Answer from the drawing. Dimensions are ordinates in mm from the lowest x, y and z of the part. A direction names the side the tool comes from. Give positions to 0.01 mm unless a question says otherwise; leave off trailing zeros. Order: outer loops, then holes, each group sorted by start corner. A loop starts at its lowest first (then second) coordinate and runs counter-clockwise, first axis right, second up. Notation, with made-up numbers: (49, 60) - (87, 60) arc R20 ccw to (87, 68) - close; hole circle Ø4 at (89.5, 88). An arc over 180 degrees is marked (long way). Use a Markdown table: item, result. Add a question column.
1) Find section D-D, the plane y = 87. Determine the outline of the cut face in (x, z).
2) Flat-ended cylindrical pins translate along their axes: pin 1 (5.5 mm diameter, centred on y = 111.5, z = 12, fed in from +X); pin 2 (9 mm diameter, centred on x = 9, y = 117, fed in from -Z); pin 3 (4 mm diameter, centred on x = 4.5, z = 4, fed in from +Y). Find the tip coordinate at first contact, or state that the pin passes through.
3) Find section B-B, the plane x = 10. Determine the outline of the cut face in (y, z).
4) Straight lines are drawn through the part: line 1 (Y direction, x = 1, z = 10); line 2 (Z direction, x = 0.75, y = 10). For each, find the intervals that lie inside material, in ascending order.
5) For the marked faces 1 and 2, determine the directions among +Z, -Z, +X, -X, +Y, -Y from which every point of the face is accessible in a straight line to the end or side of a thin tool.
6) Find section C-C, the plane z = 10. Determine the outline of the cut face in (x, y).
7) Find section A-A, the plane y = 10. Determine the outline of the cut face in (x, z), plus the area to 4 significant figures.
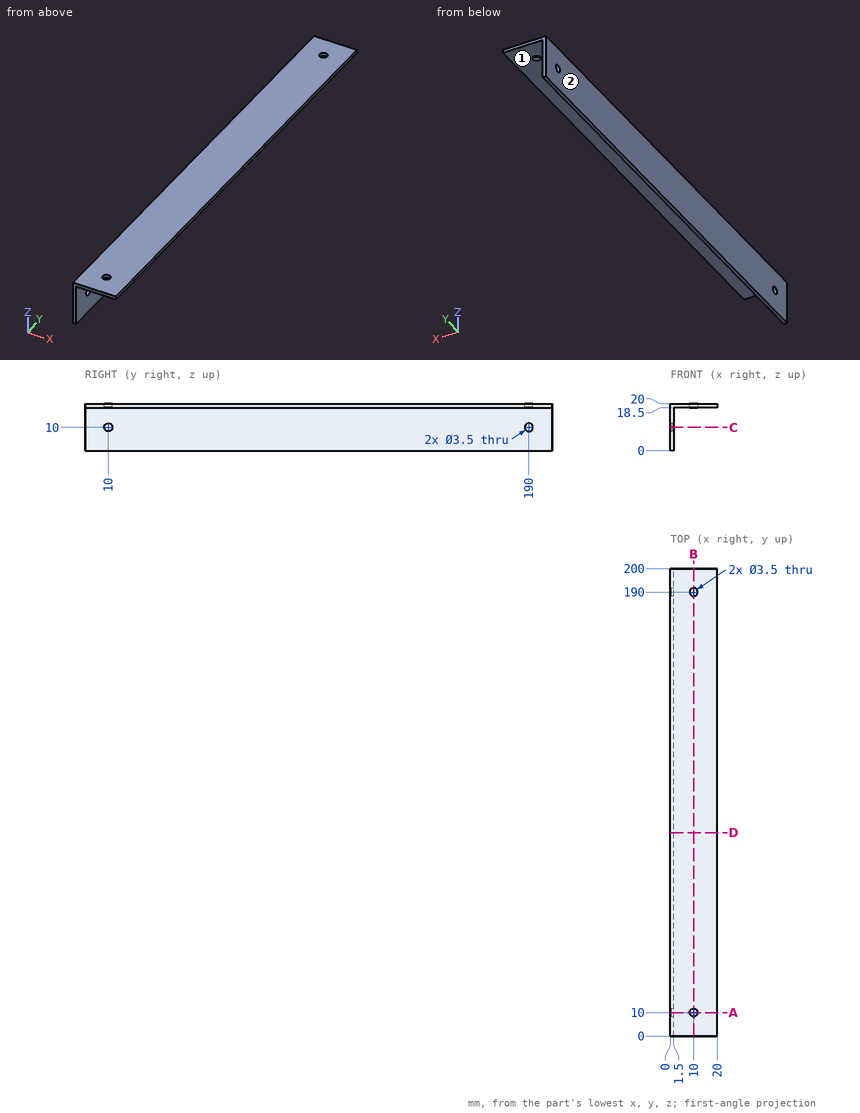
The answers:
| question | item | result |
|---|---|---|
| 1 | outline | (0, 0) - (1.5, 0) - (1.5, 18.5) - (20, 18.5) - (20, 20) - (0, 20) - close |
| 2 | pin 1 | x = 1.5 |
| 2 | pin 2 | z = 18.5 |
| 2 | pin 3 | through |
| 3 | outline | (0, 18.5) - (8.25, 18.5) - (8.25, 20) - (0, 20) - close; (11.75, 18.5) - (188.25, 18.5) - (188.25, 20) - (11.75, 20) - close; (191.75, 18.5) - (200, 18.5) - (200, 20) - (191.75, 20) - close |
| 4 | line 1 | 0 to 8.25, 11.75 to 188.25, 191.75 to 200 |
| 4 | line 2 | 0 to 8.25, 11.75 to 20 |
| 5 | face 1 | -Z, +X, +Y, -Y |
| 5 | face 2 | +Z, -Z, -X, +Y, -Y |
| 6 | outline | (0, 0) - (1.5, 0) - (1.5, 8.25) - (0, 8.25) - close; (0, 11.75) - (1.5, 11.75) - (1.5, 188.25) - (0, 188.25) - close; (0, 191.75) - (1.5, 191.75) - (1.5, 200) - (0, 200) - close |
| 7 | outline | (0, 0) - (1.5, 0) - (1.5, 8.25) - (0, 8.25) - close; (0, 11.75) - (1.5, 11.75) - (1.5, 18.5) - (8.25, 18.5) - (8.25, 20) - (0, 20) - close; (11.75, 18.5) - (20, 18.5) - (20, 20) - (11.75, 20) - close |
| 7 | area | 47.25 mm2 |
